Here's how the part is built. I have some questions about the finished solid (model axes, mm). Give positions to 0.01 mm unless a question says otherwise; leave off trailing zeros. Write each loop counter-clockwise with the first axis right and the second up, starting at its lowest first coordinate (ties: lowest second). Pieces come first, ordered by that corner, then holes. Notation, with made-up numbers: (-23, -16.75) - (36, -16.75) arc R23 cw to (36, 19.25) - close; hole circle Ø9 at (73, 17). An arc over 180 degrees is marked (long way). Use one line per item in the form item = value. Start each with the question number.
from build123d import *

# Parameters (mm, degrees)
SKETCH1_W           = 76.2
SKETCH1_H           = 6.35
BOSS_EXTRUDE1_DEPTH = 114.3
CUT_EXTRUDE1_DEPTH  = 7.35


with BuildPart() as part:
    # Sketch1 → Boss-Extrude1 (new body)
    with BuildSketch(Plane(origin=(0, 0, 0), x_dir=(1, 0, 0), z_dir=(0, 1, 0))):
        with Locations((38.1, 3.175)):
            Rectangle(SKETCH1_W, SKETCH1_H)
    extrude(amount=BOSS_EXTRUDE1_DEPTH)

    # Sketch2 → Cut-Extrude1 (cut, through all)
    with BuildSketch(Plane.XY):
        with BuildLine():
            Line((48.41875, 87.3125), (48.41875, 76.99375))
            ThreePointArc((48.41875, 76.99375), (38.1, 66.675), (27.78125, 76.99375))
            Line((27.78125, 76.99375), (27.78125, 87.3125))
            ThreePointArc((27.78125, 87.3125), (38.1, 97.63125), (48.41875, 87.3125))
        make_face()
    extrude(amount=-CUT_EXTRUDE1_DEPTH, mode=Mode.SUBTRACT)


solid = part.part
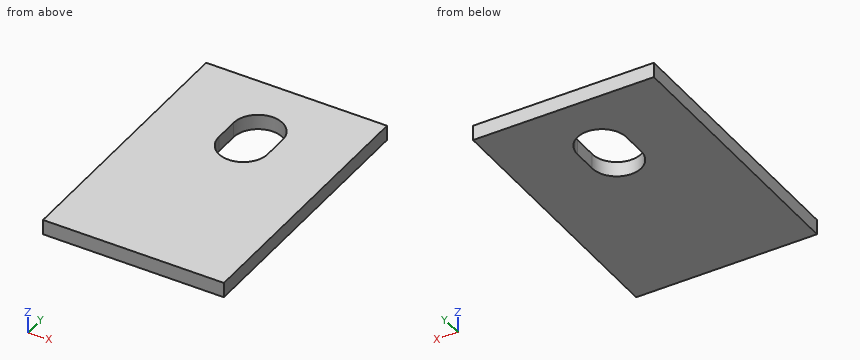
1. I want a section at C-C, the plane z = -1.5. List the corners of the cut face in (x, y) for me, then the cut area to 3 significant figures.
2. I want a section at A-A, the plane y = 83. List the corners of the cut face in (x, z) for me.
3. Please list where these lines run through material, in increasing order: line 1 (Y direction, x = 30.5, z = -1); line 2 (Y direction, x = 43, z = -2); line 3 (X direction, y = 81, z = -1.75).
4. I want a section at B-B, the plane x = 38.1. List the corners of the cut face in (y, z) for me (3 decimals).
Result sheet:
q1.outline = (0, 0) - (76.2, 0) - (76.2, 114.3) - (0, 114.3) - close; hole (27.78, 76.99) arc R10.32 ccw to (48.42, 76.99) - (48.42, 87.31) arc R10.32 ccw to (27.78, 87.31) - close
q1.area = 8,160 mm2
q2.outline = (0, -6.35) - (27.78, -6.35) - (27.78, 0) - (0, 0) - close; (48.42, -6.35) - (76.2, -6.35) - (76.2, 0) - (48.42, 0) - close
q3.line_1 = 0 to 70.01, 94.29 to 114.3
q3.line_2 = 0 to 67.91, 96.39 to 114.3
q3.line_3 = 0 to 27.78, 48.42 to 76.2
q4.outline = (0, -6.35) - (66.675, -6.35) - (66.675, 0) - (0, 0) - close; (97.631, -6.35) - (114.3, -6.35) - (114.3, 0) - (97.631, 0) - close
